Build history of the part. All positions in model axes, mm. A direction names the side the tool comes from. Coordinates: 2 decimals unless noted, no trailing zeros. Write each loop counter-clockwise with the first axis right and the second up, starting at its lowest first coordinate (ties: lowest second). Pieces come first, ordered by that corner, then holes.
```python
from build123d import *

# Parameters (mm, degrees)
SKETCH1_R           = 2.8702
BOSS_EXTRUDE1_DEPTH = 3.5052
SKETCH2_R           = 1.7526
BOSS_EXTRUDE2_DEPTH = 19.05
SKETCH3_OUTSIDE_W   = 12.534
SKETCH3_OUTSIDE_H   = 12.534
SKETCH3_OUTSIDE_R   = 1.35255
CUT_EXTRUDE1_DEPTH  = 19.05
CUT_EXTRUDE2_DEPTH  = 1.6256


with BuildPart() as part:
    # Sketch1 → Boss-Extrude1 (new body)
    with BuildSketch(Plane.XY):
        Circle(SKETCH1_R)
    extrude(amount=BOSS_EXTRUDE1_DEPTH)

    # Sketch2 → Boss-Extrude2 (add)
    with BuildSketch(Plane(origin=(0, 0, 0), x_dir=(-1, 0, 0), z_dir=(0, 0, -1))):
        with Locations(Location((0, 0, 0), (0, 0, 180))):
            Circle(SKETCH2_R)
    extrude(amount=BOSS_EXTRUDE2_DEPTH)

    # Sketch3 outside → Cut-Extrude1 (cut)
    with BuildSketch(Plane(origin=(0, 0, -19.05), x_dir=(-1, 0, 0), z_dir=(0, 0, -1))):
        Rectangle(SKETCH3_OUTSIDE_W, SKETCH3_OUTSIDE_H)
        Circle(SKETCH3_OUTSIDE_R, mode=Mode.SUBTRACT)
    extrude(amount=-CUT_EXTRUDE1_DEPTH, mode=Mode.SUBTRACT)

    # Sketch4 → Cut-Extrude2 (cut)
    with BuildSketch(Plane.XY.offset(3.5052)):
        Polygon((0.801975608, 1.3890625), (-0.801975608, 1.3890625), (-1.603951217, 0), (-0.801975608, -1.3890625), (0.801975608, -1.3890625), (1.603951217, 0), align=None)
    extrude(amount=-CUT_EXTRUDE2_DEPTH, mode=Mode.SUBTRACT)


solid = part.part
```
1. 3-axis set-ups, long thin cutter, end or side, ignore diameter. For faces 1 (the face through (-2.278, -1.746, 1.728)), 2 (the face through (0, 1.389, 3)): which of +Z, -Z, +X, -X, +Y, -Y reach the whole face in a straight line?
Computed values:
face 1: +Z, -Z
face 2: +Z
2. Saw through at D-D on y = -2. List the corners of the cut face in (x, z).
Computed values:
outline: (-2.06, 0) - (2.06, 0) - (2.06, 3.51) - (-2.06, 3.51) - close
3. Saw through at A-A on x = 0. List the corners of the cut face in (y, z).
Computed values:
outline: (-2.87, 0) - (-1.35, 0) - (-1.35, -19.05) - (1.35, -19.05) - (1.35, 0) - (2.87, 0) - (2.87, 3.51) - (1.39, 3.51) - (1.39, 1.88) - (-1.39, 1.88) - (-1.39, 3.51) - (-2.87, 3.51) - close
4. Mould opens along X. For faces 3 (the face through (0, 0, -19.05)), 4 (the face through (0, 0, 1.88)), 5 (the face through (-1.29, 0.41, -9.66)) say: +X half, -X half, draft (parallel to the pull), parting line (faces both ways), or undercut.
Computed values:
face 3: draft
face 4: undercut
face 5: parting line
5. Flat gauge pin, fed straight in: pin 1 (1 mm diameter, centred on x = -0.5, z = -9.5, fed in from -Y). Where does the tip first touch, or does it go through?
Computed values:
pin 1: stops at y = -1.35
6. Saw through at C-C on y = 1.05. List the corners of the cut face in (x, z), plus the area to 3 significant figures.
Computed values:
outline: (-2.67, 0) - (-0.85, 0) - (-0.85, -19.05) - (0.85, -19.05) - (0.85, 0) - (2.67, 0) - (2.67, 3.51) - (1, 3.51) - (1, 1.88) - (-1, 1.88) - (-1, 3.51) - (-2.67, 3.51) - close
area: 48.0 mm2
7. Saw through at B-B on z = -13.5. List the corners of the cut face in (x, y), plus the area to 3 significant figures.
Computed values:
outline: circle Ø2.71 at (0, 0)
area: 5.75 mm2
8. Probe line 1 along Z through (x, y) = (0.1, 1.6); line 2 along Z through (x, y) = (1.45, 0.1); line 3 along Y through (x, z) = (0.25, -8). List the from-to ranges inside material, lowest first.
Computed values:
line 1: z = 0 to 3.51
line 2: z = 0 to 1.88
line 3: y = -1.33 to 1.33
